The model under review builds one solid part; all positions refer to its coordinate system, in mm. Give positions to 0.01 mm unless a question says otherwise; leave off trailing zeros. Order: outer loops, then holes, each group sorted by start corner. A loop starts at its lowest first (then second) coordinate and runs counter-clockwise, first axis right, second up. Notation, with made-up numbers: (32.5, 6) -> (70.5, 6) arc R29 cw to (70.5, 35) -> close; hole circle Ø3 at (12, 60.5). An arc over 180 degrees is marked (long way). Use one line per item in the form item = value.
Autodesk Inventor part; units mm, degrees
ref_plane "YZ Plane" through (0, 0, 0) normal (1, 0, 0) x (0, 1, 0)
ref_plane "XZ Plane" through (0, 0, 0) normal (0, 1, 0) x (-1, 0, 0)
ref_plane "XY Plane" through (0, 0, 0) normal (0, 0, 1) x (1, 0, 0)
sketch "Sketch2" plane through (0, 0, 0) normal (0, 0, 1) x (1, 0, 0)
  line L0 (0, 297.5) -> (0, -297.5) construction
  line L1 (-402.5, 0) -> (402.5, 0) construction
  line L2 (-287.5, 212.5) -> (287.5, 212.5)
  line L3 (287.5, 212.5) -> (287.5, -212.5)
  line L4 (287.5, -212.5) -> (-287.5, -212.5)
  line L5 (-287.5, -212.5) -> (-287.5, 212.5)
  point P0 (0, 0)
  dimension "d0" = 425
  dimension "d1" = 575
extrude "Extrusion1" add sketch "Sketch2" along normal blind 2
sketch "Sketch3" plane through (0, 0, 2) normal (0, 0, 1) x (1, 0, 0)
  line L0 (287.5, 212.5) -> (-287.5, 212.5) construction
  line L1 (-287.5, 212.5) -> (-287.5, -212.5) construction
  line L2 (-287.5, -212.5) -> (287.5, -212.5) construction
  line L3 (287.5, -212.5) -> (287.5, 212.5) construction
  line L4 (287.5, 212.5) -> (-287.5, 212.5)
  line L5 (287.5, 212.5) -> (265.5, 212.5)
  line L6 (265.5, 212.5) -> (265.5, 142.5)
  line L7 (265.5, 142.5) -> (287.5, 142.5)
  line L8 (287.5, 142.5) -> (287.5, 212.5)
  line L9 (287.5, -212.5) -> (265.5, -212.5)
  line L10 (265.5, -212.5) -> (265.5, -142.5)
  line L11 (265.5, -142.5) -> (287.5, -142.5)
  line L12 (287.5, -142.5) -> (287.5, -212.5)
  point P0 (0, 0)
  dimension "d4" = 22
  dimension "d5" = 70
  dimension "d6" = 70
extrude "Extrusion2" cut sketch "Sketch3" against normal blind 2
sketch "Sketch4" plane through (0, 0, 2) normal (0, 0, 1) x (1, 0, 0)
  line L0 (265.5, 142.5) -> (265.5, 212.5) construction
  line L1 (265.5, 212.5) -> (-287.5, 212.5) construction
  line L2 (-287.5, 212.5) -> (-287.5, -212.5) construction
  line L3 (-287.5, -212.5) -> (265.5, -212.5) construction
  line L4 (265.5, -212.5) -> (265.5, -142.5) construction
  line L5 (265.5, -142.5) -> (287.5, -142.5) construction
  line L6 (287.5, -142.5) -> (287.5, 142.5) construction
  line L7 (287.5, 142.5) -> (265.5, 142.5) construction
  line L8 (265.5, 142.5) -> (265.5, 212.5) construction
  line L9 (265.5, 200) -> (-287.5, 200) construction
  line L10 (-287.5, 212.5) -> (265.5, 212.5) construction
  line L11 (-268.0097, 212.5) -> (-268.0097, -212.5) construction
  line L12 (-287.5, -212.5) -> (265.5, -212.5) construction
  line L13 (-287.5, -200) -> (265.5, -200) construction
  point P0 (0, 0)
  point P1 (187.5, 200)
  point P2 (-187.5, 200)
  point P3 (-187.5, -200)
  point P4 (187.5, -200)
  point P5 (-185.9119, -200.0708)
  dimension "d9" = 12.5
  dimension "d10" = 12.5
  dimension "d11" = 100
  dimension "d12" = 100
  dimension "d13" = 100
  dimension "d14" = 100
hole "Hole1" at (-187.5, 200, 2) at (187.5, 200, 2) at (187.5, -200, 2) at (-185.9119, -200.0708, 2) direction (0, 0, -1) diameter 6 depth 10 tip angle 118
properties part number "Top_Cover_V1"
1. For L1, parallel to X at y = -200, z = 1.65; L2, parallel to X at y = 200, z = 0.6; L3, parallel to Y at x = -187.5, z = 1.1, list the stretches that pass through material, from the lowest coordinate up.
Values:
L1 = -287.5 to -188.91, -182.91 to 184.5, 190.5 to 265.5
L2 = -287.5 to -190.5, -184.5 to 184.5, 190.5 to 265.5
L3 = -212.5 to -202.62, -197.53 to 197, 203 to 212.5
2. For pin 1 Ø5 at (x, y) = (187.5, -200) entering from -Z; pin 2 Ø0.6 at (y, z) = (166, 0.5) entering from +X; pin 3 Ø1 at (x, z) = (275, 0.5) entering from +Y; pin 4 Ø9.5 at (x, y) = (187.5, 200) entering from +Z, all flat-tipped, find the tip position at first contact; note any pin that passes through.
Values:
pin_1 = through
pin_2 = 265.5
pin_3 = 142.5
pin_4 = 2
3. Add section A-A on y = -156. Give the boundary of the cut face in (x, z).
Values:
outline = (-287.5, 0) -> (265.5, 0) -> (265.5, 2) -> (-287.5, 2) -> close
